```python
from build123d import *

# Parameters (mm, degrees)
EXTRUDE_1_DEPTH          = 3
SKETCH_2_W               = 10.886343204
SKETCH_2_H               = 8.708921112
CUT_EXTRUDE_1_DEPTH      = 1
CUT_EXTRUDE_1_DEPTH_BACK = 4
SKETCH_3_R               = 1.9
CUT_EXTRUDE_2_DEPTH      = 1
CUT_EXTRUDE_2_DEPTH_BACK = 4
SKETCH_4_R               = 1.49
CUT_EXTRUDE_3_DEPTH      = 1
CUT_EXTRUDE_3_DEPTH_BACK = 4
SKETCH_5_W               = 49.113656796
SKETCH_5_H               = 0.5
EXTRUDE_2_DEPTH          = 3


with BuildPart() as part:
    # Эскиз1 → Бобышка-Вытянуть1 (new body)
    with BuildSketch(Plane.XY):
        with BuildLine():
            Line((45.301358773, 22.383876488), (45.301358773, -1.452573816))
            Line((45.301358773, -1.452573816), (53, 0))
            Line((53, 0), (53.661481565, 0.375))
            Line((53.661481565, 0.375), (105.301358773, 0.375))
            ThreePointArc((105.301358773, 0.375), (106.2209108, 0.982031719), (106.024068331, 2.066151861))
            Line((106.024068331, 2.066151861), (86.593533576, 22.383876488))
            Line((86.593533576, 22.383876488), (45.301358773, 22.383876488))
        make_face()
    extrude(amount=EXTRUDE_1_DEPTH)

    # Эскиз2 → Вырез-Вытянуть1 (cut, two sides)
    with BuildSketch(Plane.XY.offset(3)) as cut_extrude_1_sk:
        with Locations((50.744530375, -1.111990753)):
            Rectangle(SKETCH_2_W, SKETCH_2_H)
    extrude(amount=CUT_EXTRUDE_1_DEPTH, mode=Mode.SUBTRACT)
    extrude(cut_extrude_1_sk.sketch, amount=-CUT_EXTRUDE_1_DEPTH_BACK, mode=Mode.SUBTRACT)

    # Эскиз3 → Вырез-Вытянуть2 (cut, two sides)
    with BuildSketch(Plane.XY.offset(3)) as cut_extrude_2_sk:
        with Locations((52.593533576, 10.375)):
            Circle(SKETCH_3_R)
        with Locations((72.593533576, 10.375)):
            Circle(SKETCH_3_R)
        with Locations((92.593533576, 10.375)):
            Circle(SKETCH_3_R)
    extrude(amount=CUT_EXTRUDE_2_DEPTH, mode=Mode.SUBTRACT)
    extrude(cut_extrude_2_sk.sketch, amount=-CUT_EXTRUDE_2_DEPTH_BACK, mode=Mode.SUBTRACT)

    # Эскиз4 → Вырез-Вытянуть3 (cut, two sides)
    with BuildSketch(Plane.XY.offset(3)) as cut_extrude_3_sk:
        with Locations((92.705183178, 2.375)):
            Circle(SKETCH_4_R)
        with Locations((70.705183178, 2.375)):
            Circle(SKETCH_4_R)
    extrude(amount=CUT_EXTRUDE_3_DEPTH, mode=Mode.SUBTRACT)
    extrude(cut_extrude_3_sk.sketch, amount=-CUT_EXTRUDE_3_DEPTH_BACK, mode=Mode.SUBTRACT)

    # Эскиз5 → Бобышка-Вытянуть2 (add)
    with BuildSketch(Plane.XY.offset(3)):
        with Locations((80.744530375, 0.125)):
            Rectangle(SKETCH_5_W, SKETCH_5_H)
    extrude(amount=-EXTRUDE_2_DEPTH)


solid = part.part
```
Verification items for the finished model (mm, model axes). A direction names the side the tool comes from. Give positions to 0.01 mm unless a question says otherwise; leave off trailing zeros. Order: outer loops, then holes, each group sorted by start corner. A loop starts at its lowest first (then second) coordinate and runs counter-clockwise, first axis right, second up. Notation, with made-up numbers: M 69,41.5 L 127,41.5 A28 ccw 127,63.5 Z; hole C 27.25,57.25 d2. An arc over 180 degrees is marked long. Return JSON: item names as keys, results as strings. Group by question number.
1) Go/stop test with a flat-tipped pin: pin 1 Ø0.9 at (x, z) = (50.5, 1) entering from -Y. Record where the tip stops, or that it passes through.
2) Access from +Z, -Z, +X, -X, +Y, -Y to the whole of each face (thin tool, end or side, straight path). Record for faces 1 (the face through (69, 11, 3)), 2 (the face through (56.188, 2, 2)).
3) Scan lines: line 1 (Y direction, x = 71.5, z = 0.4) (3 decimals); line 2 (Y direction, x = 93.5, z = 0.6) (3 decimals); line 3 (Y direction, x = 91, z = 1.45) (3 decimals). Record each from-to range of solid material in increasing order.
4) Mould release check, pull along X, two halves, no side actions. Record for faces 3 (the face through (51, 3.242, 2)), 4 (the face through (70.695, 10.459, 1.521)), 5 (the face through (45.301, 13, 1)), 6 (the face through (54.35, 9.65, 1.52)): pulls with the +X half, pulls with the -X half, needs draft (parallel to the pull), parting line crosses it, or undercut.
5) Section check C-C on x = 93.5. Record the cut outline in (y, z) (3 decimals), and give its area (3 significant figures).
6) Section check D-D on y = 5.25. Record the cut outline in (x, z).
7) Section check A-A on y = 11. Record the cut outline in (x, z), and give its area (3 significant figures).
8) Section check B-B on z = 0.45. Record the cut outline in (x, y) (3 decimals).
Answer block:
{
 "1": {"pin 1": "stops at y = 3.24"},
 "2": {"face 1": "+Z, +X, -X, +Y, -Y", "face 2": "+Z, -Z, -X, -Y"},
 "3": {"line 1": "y = -0.125 to 1.115, 3.635 to 8.821, 11.929 to 22.384", "line 2": "y = -0.125 to 1.115, 3.635 to 8.705, 12.045 to 15.162", "line 3": "y = -0.125 to 9.34, 11.41 to 17.776"},
 "4": {"face 3": "needs draft", "face 4": "undercut", "face 5": "pulls with the -X half", "face 6": "undercut"},
 "5": {"outline": "M -0.125,0 L 1.115,0 L 1.115,3 L -0.125,3 Z; M 3.635,0 L 8.705,0 L 8.705,3 L 3.635,3 Z; M 12.045,0 L 15.162,0 L 15.162,3 L 12.045,3 Z", "area": "28.3 mm^2"},
 "6": {"outline": "M 45.3,0 L 102.98,0 L 102.98,3 L 45.3,3 Z"},
 "7": {"outline": "M 45.3,0 L 50.8,0 L 50.8,3 L 45.3,3 Z; M 54.39,0 L 70.8,0 L 70.8,3 L 54.39,3 Z; M 74.39,0 L 90.8,0 L 90.8,3 L 74.39,3 Z; M 94.39,0 L 97.48,0 L 97.48,3 L 94.39,3 Z", "area": "124 mm^2"},
 "8": {"outline": "M 45.301,3.242 L 56.188,3.242 L 56.188,-0.125 L 105.301,-0.125 L 105.301,0.375 A1 ccw 106.024,2.066 L 86.594,22.384 L 45.301,22.384 Z; hole C 52.594,10.375 d3.8; hole C 70.705,2.375 d2.98; hole C 72.594,10.375 d3.8; hole C 92.594,10.375 d3.8; hole C 92.705,2.375 d2.98"}
}
